CAD build for the part. Positions are in the model's coordinates, mm. Face numbers are marked on the shaded views. A direction names the side the tool comes from. Round coordinates to 2 decimals unless told otherwise and drop trailing zeros. Loops run counter-clockwise (first coordinate to the right, second up) from the corner with the lowest first, then second, coordinate; pieces in that order, holes last.
```python
from build123d import *

# Parameters (mm, degrees)
F0_W      = 58
F0_H      = 70
F4_DEPTH  = 19
F3_R      = 2.5
F5_DEPTH  = 14
F2_R      = 4
F6_DEPTH  = 5
F7_DEPTH  = 19
F8_DEPTH  = 5
F9_R      = 2.75
F10_DEPTH = 19
F12_DEPTH = 4
F13_W     = 26
F13_H     = 19
F14_DEPTH = 19
F15_R     = 2
F16_R     = 4.375
F16_R_2   = 2.75
F17_DEPTH = 5.5


with BuildPart() as f4:
    # F0 (on Top) → F4 (new body)
    with BuildSketch(Plane.XY):
        Rectangle(F0_W, F0_H)
    extrude(amount=F4_DEPTH)

    # F3 (on Top) → F5 (cut)
    with BuildSketch(Plane.XY):
        with Locations((-21.9419958555, 25.0643808395)):
            Circle(F3_R)
    extrude(amount=F5_DEPTH, mode=Mode.SUBTRACT)

    # F2 (on Top) → F6 (cut)
    with BuildSketch(Plane.XY):
        with Locations((-21.9419958555, 25.0643808395)):
            Circle(F2_R)
    extrude(amount=F6_DEPTH, mode=Mode.SUBTRACT)

    # F3 (on Top) → F7 (cut)
    with BuildSketch(Plane.XY):
        with Locations((-21.9419958555, 25.0643808395)):
            Circle(F3_R)
        with Locations((22.0838580281, 24.9406788498)):
            Circle(F3_R)
        with Locations((-21.9535976648, -25.1581091434)):
            Circle(F3_R)
        with Locations((22.0838580281, -25.1581091434)):
            Circle(F3_R)
    extrude(amount=F7_DEPTH, mode=Mode.SUBTRACT)

    # F2 (on Top) → F8 (cut)
    with BuildSketch(Plane.XY):
        with Locations((-21.9419958555, 25.0643808395)):
            Circle(F2_R)
        with Locations((-21.9535976648, -25.1581091434)):
            Circle(F2_R)
        with Locations((22.0838580281, -25.1581091434)):
            Circle(F2_R)
        with Locations((22.0838580281, 24.9406788498)):
            Circle(F2_R)
    extrude(amount=F8_DEPTH, mode=Mode.SUBTRACT)

    # F9 (on Top) → F10 (cut)
    with BuildSketch(Plane.XY):
        with Locations((17.5465345383, 8.045819588)):
            Circle(F9_R)
        with Locations((-17.3794273287, -8.1804059446)):
            Circle(F9_R)
    extrude(amount=F10_DEPTH, mode=Mode.SUBTRACT)

    # F11 (on face) → F12 (cut)
    with BuildSketch(Plane(origin=(0, 0, 0), x_dir=(1, 0, 0), z_dir=(0, 0, -1))):
        Polygon((-15.0014997318, 12.5717974553), (-20.001031324, 12.5033587326), (-22.4415274477, 8.1394180054), (-19.8824919791, 3.8439160009), (-14.8829603869, 3.9123547236), (-12.4424642633, 8.2762954508), align=None)
        Polygon((19.4248843713, -12.627403312), (22.5651466247, -8.7365482672), (20.7656984402, -4.0715738588), (15.8259880023, -3.2974544952), (12.6857257488, -7.1883095399), (14.4851739333, -11.8532839484), align=None)
    extrude(amount=-F12_DEPTH, mode=Mode.SUBTRACT)

    # F13 (on Top) → F14 (cut)
    with BuildSketch(Plane.XY):
        with Locations((-0.0902060419, 25.5731031678)):
            Rectangle(F13_W, F13_H)
        with Locations((-0.0902060419, -25.5731031678)):
            Rectangle(F13_W, F13_H)
    extrude(amount=F14_DEPTH, mode=Mode.SUBTRACT)

    # F15
    f15_edges = [f4.edges().sort_by_distance(p)[0] for p in [
        (-13.090206, 25.536552, 0),
        (-0.090206, 16.073103, 0),
        (12.909794, 25.536552, 0),
        (-21.045103, 35, 0),
        (-29, 0, 0),
        (-21.045103, -35, 0),
        (-13.090206, -25.536552, 0),
        (-0.090206, -16.073103, 0),
        (12.909794, -25.536552, 0),
        (20.954897, -35, 0),
        (29, 0, 0),
        (20.954897, 35, 0),
        (-13.090206, 35, 9.5),
        (-13.090206, 16.073103, 9.5),
        (12.909794, 35, 9.5),
        (29, 35, 9.5),
        (-29, 35, 9.5),
        (-21.045103, 35, 19),
        (-13.090206, 25.536552, 19),
        (-0.090206, 16.073103, 19),
        (20.954897, 35, 19),
        (29, 0, 19),
        (29, -35, 9.5),
        (12.909794, 25.536552, 19),
        (-29, -35, 9.5),
        (-29, 0, 19),
        (-13.090206, -35, 9.5),
        (12.909794, -35, 9.5),
        (12.909794, -25.536552, 19),
        (12.909794, -16.073103, 9.5),
        (20.954897, -35, 19),
        (-21.045103, -35, 19),
        (-0.090206, -16.073103, 19),
        (-13.090206, -25.536552, 19),
        (-13.090206, -16.073103, 9.5),
        (12.909794, 16.073103, 9.5),
    ]]
    fillet(f15_edges, radius=F15_R)

    # F16 (on face) → F17 (cut)
    with BuildSketch(Plane.XY.offset(19)):
        with Locations((-17.3794273287, -8.1804059446)):
            Circle(F16_R)
        with Locations((-17.3794273287, -8.1804059446)):
            Circle(F16_R_2, mode=Mode.SUBTRACT)
        with Locations((17.5465345383, 8.045819588)):
            Circle(F16_R)
        with Locations((17.5465345383, 8.045819588)):
            Circle(F16_R_2, mode=Mode.SUBTRACT)
    extrude(amount=-F17_DEPTH, mode=Mode.SUBTRACT)


solid = f4.part
```
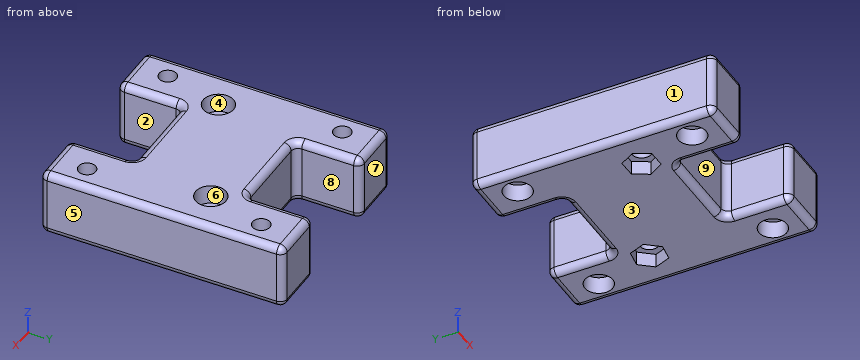
Item 1: Probe line 1 (X direction, y = -19.5, z = 7.75); line 2 (Y direction, x = -19.5, z = 4.25); line 3 (X direction, y = 23.5, z = 12.75). List the from-to ranges inside material, lowest first.
Answers follow:
line 1: x = -29 to -13.09, 12.91 to 29
line 2: y = -35 to -28.32, -22 to -9.93, -6.43 to 21.9, 28.23 to 35
line 3: x = -29 to -23.89, -19.99 to -13.09, 12.91 to 20.04, 24.13 to 29
Item 2: 3-axis set-ups, long thin cutter, end or side, ignore diameter. For the marked faces 5, 6, 7, 8 and 9: which of +Z, -Z, +X, -X, +Y, -Y reach the whole face in a straight line?
Answers follow:
face 5: +Z, -Z, +X, +Y, -Y
face 6: +Z
face 7: +Z, -Z, +X, -X, +Y
face 8: +Z, -Z, +Y
face 9: +Z, -Z, -Y
Item 3: Cut at A-A, the plane y = -26.5. State how many separate pieces and enclosed holes the cut face has, plus the area to 3 significant figures.
Answers follow:
separate pieces: 4
enclosed holes: 0
area: 408 mm2
Item 4: Flat gauge pins, fed straight in: P1, Ø7, axis at x = 17.55, y = 8.05, coming from the -Z side; P2, Ø6.5, axis at x = 22.08, y = 24.94, coming from the -Z side; P3, Ø3.5, axis at x = -17.38, y = -8.18, coming from the +Z side; P4, Ø1, axis at x = -2.5, z = 2, coming from the +Y side. Where does each tip first touch, or does it go through?
Answers follow:
P1: stops at z = 4
P2: stops at z = 5
P3: passes through
P4: stops at y = 16.07
Item 5: Two-plate mould, pull along X, no slides. Class the marked faces 1, 2, 3 and 4: released by +X, released by -X, zero draft, split by the parting line, or undercut.
Answers follow:
face 1: released by -X
face 2: undercut
face 3: zero draft
face 4: undercut
Item 6: Cut at B-B, the plane x = -2. Give the cut face in (y, z), plus the area to 3 significant figures.
Answers follow:
outline: (-16.07, 2) arc R2 ccw to (-14.07, 0) - (14.07, 0) arc R2 ccw to (16.07, 2) - (16.07, 17) arc R2 ccw to (14.07, 19) - (-14.07, 19) arc R2 ccw to (-16.07, 17) - close
area: 607 mm2
Item 7: Cut at C-C, the plane x = -16. Give the cut face in (y, z), plus the area to 3 significant figures.
Answers follow:
outline: (-35, 2) arc R2 ccw to (-33, 0) - (-12.56, 0) - (-12.56, 4) - (-10.56, 4) - (-10.56, 13.5) - (-12.33, 13.5) - (-12.33, 19) - (-33, 19) arc R2 ccw to (-35, 17) - close; (-5.8, 4) - (-3.9, 4) - (-3.9, 0) - (33, 0) arc R2 ccw to (35, 2) - (35, 17) arc R2 ccw to (33, 19) - (-4.03, 19) - (-4.03, 13.5) - (-5.8, 13.5) - close
area: 1,200 mm2
